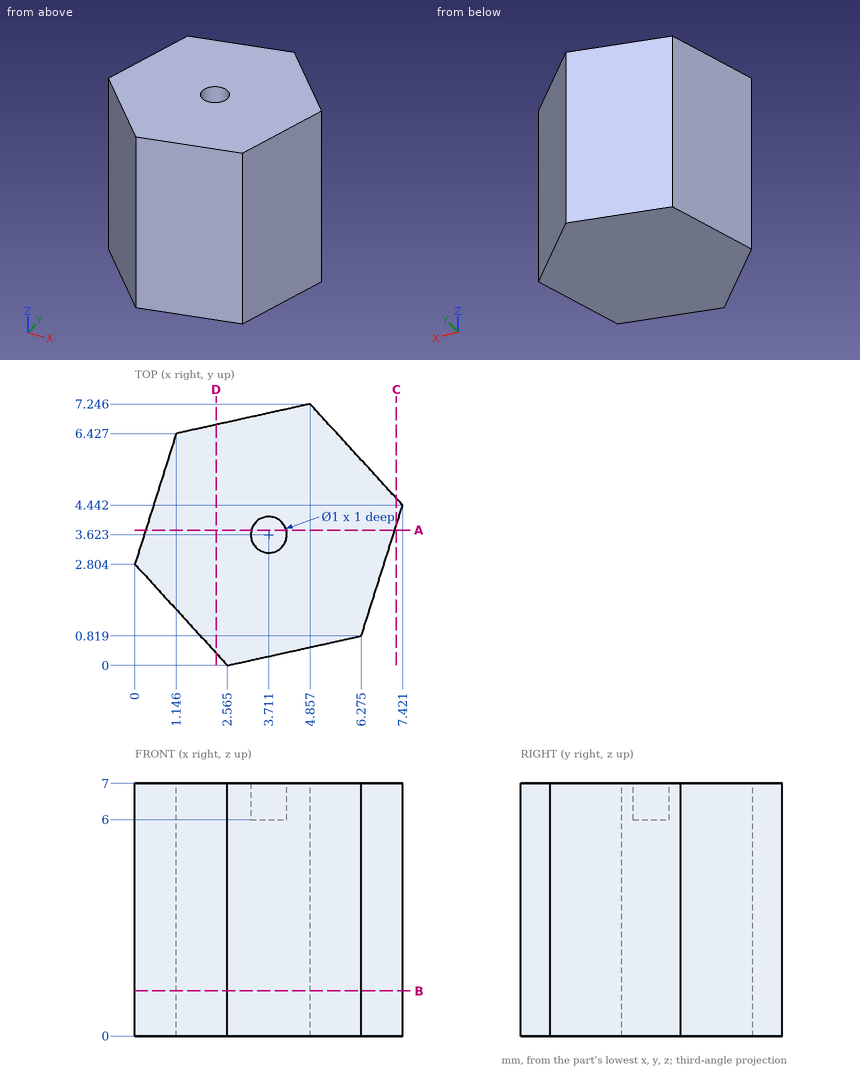
Could you check a few things on this drawing? It's one solid part, dimensions in mm from its lowest x, y, z. Give positions to 0.01 mm unless a question says otherwise; leave off trailing zeros. Write each loop counter-clockwise with the first axis right and the second up, starting at its lowest first coordinate (ties: lowest second). Pieces come first, ordered by that corner, then holes.
(1) Imagine slicing it at C-C, the plane x = 7.25. Write out the boundary of the cut face in (y, z).
Output values:
outline: (3.9, 0) - (4.63, 0) - (4.63, 7) - (3.9, 7) - close
(2) Imagine slicing it at A-A, the plane y = 3.75. Write out the boundary of the cut face in (x, z) (1 decimal).
Output values:
outline: (0.3, 0) - (7.2, 0) - (7.2, 7) - (4.2, 7) - (4.2, 6) - (3.2, 6) - (3.2, 7) - (0.3, 7) - close
(3) Imagine slicing it at D-D, the plane x = 2.25. Write out the boundary of the cut face in (y, z).
Output values:
outline: (0.34, 0) - (6.67, 0) - (6.67, 7) - (0.34, 7) - close
(4) If I drill on L1, parallel to Y at x = 3, z = 0.5 (1 decimal); L2, parallel to X at y = 3.25, z = 1.5 (1 decimal); L3, parallel to Y at x = 5.75, z = 4.5 (1 decimal), over which ranges is the centre line in solid material (lowest first)?
Output values:
L1: y = 0.1 to 6.8
L2: x = 0.1 to 7
L3: y = 0.7 to 6.3
(5) Will these pins go through, and if not, where does the flat tip stop? pin 1 (4 mm diameter, centred on y = 2.5, z = 3, fed in from -X); pin 2 (1.5 mm diameter, centred on y = 1.5, z = 5, fed in from -X); pin 3 (1.5 mm diameter, centred on y = 5.5, z = 1, fed in from +X).
Output values:
pin 1: stops at x = 0
pin 2: stops at x = 0.51
pin 3: stops at x = 7.14
(6) Imagine slicing it at B-B, the plane z = 1.25. Write out the boundary of the cut face in (x, y) (1 decimal), and give its area (3 significant figures).
Output values:
outline: (0, 2.8) - (2.6, 0) - (6.3, 0.8) - (7.4, 4.4) - (4.9, 7.2) - (1.1, 6.4) - close
area: 37.5 mm2
